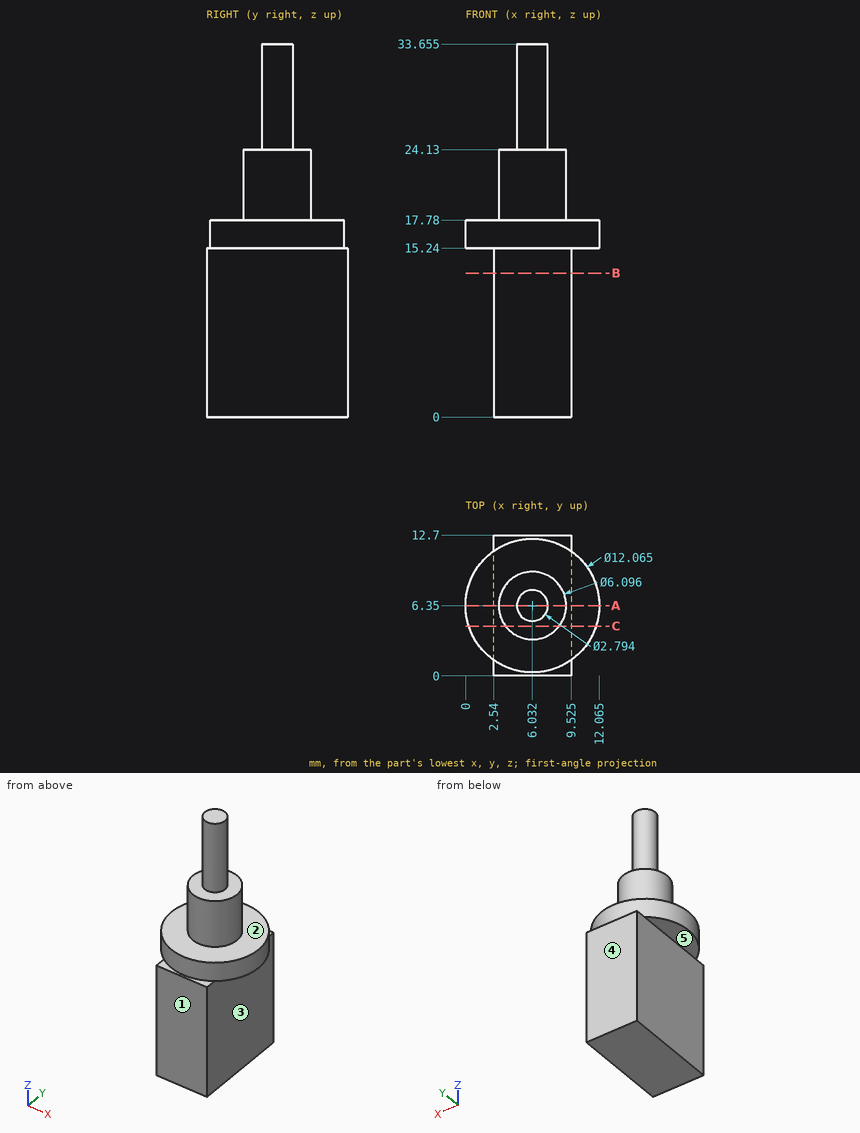
Geometry: see drawing. Coordinates: mm, zero at the bounding-box minimum. A direction names the side the tool comes from. Give positions to 0.01 mm unless a question says otherwise; leave off trailing zeros. Order: outer loops, then holes, each group sorted by start corner. A loop starts at its lowest first (then second) coordinate and runs counter-clockwise, first axis right, second up. Notation, with made-up numbers: M 24,71.25 L 82,71.25 A7 cw 82,83.25 Z; hole C 43,-32 d3. An arc over 180 degrees is marked long. Answer as a JSON object with one key per item and string values.
1. Cut plane B-B, the plane z = 13. Output: boundary loops of the cut face in (x, y) (1 decimal).
Result sheet:
{"outline": "M 2.5,0 L 9.5,0 L 9.5,12.7 L 2.5,12.7 Z"}
2. First-contact query: P1, Ø0.8, axis at x = 1.5, y = 6, coming from the -Z side; P2, Ø1.6, axis at x = 6.5, y = 1, coming from the +Z side; P3, Ø5, axis at x = 9.5, z = 15.5, coming from the -Y side; P4, Ø4, axis at y = 4.5, z = 6.5, coming from the -X side. Flat tips, straight axial feed; report the tip coordinate or a pass-through.
Result sheet:
{"P1": "z = 15.24", "P2": "z = 17.78", "P3": "y = 0", "P4": "x = 2.54"}
3. Ray query, line 1 (Z direction, x = 10, y = 6.75); line 2 (Z direction, x = 3.75, y = 10.25); line 3 (X direction, y = 5.5, z = 6) (1 decimal). Return the intervals inside material, ascending. Write a range as [from, to].
Result sheet:
{"line 1": "[15.24, 17.78]", "line 2": "[0, 17.78]", "line 3": "[2.5, 9.5]"}
4. Cut plane A-A, the plane y = 6.35. Output: boundary loops of the cut face in (x, z) (1 decimal).
Result sheet:
{"outline": "M 0,15.2 L 2.5,15.2 L 2.5,0 L 9.5,0 L 9.5,15.2 L 12.1,15.2 L 12.1,17.8 L 9.1,17.8 L 9.1,24.1 L 7.4,24.1 L 7.4,33.7 L 4.6,33.7 L 4.6,24.1 L 3,24.1 L 3,17.8 L 0,17.8 Z"}
5. Cut plane C-C, the plane y = 4.5. Output: boundary loops of the cut face in (x, z) (1 decimal).
Result sheet:
{"outline": "M 0.3,15.2 L 2.5,15.2 L 2.5,0 L 9.5,0 L 9.5,15.2 L 11.8,15.2 L 11.8,17.8 L 8.5,17.8 L 8.5,24.1 L 3.6,24.1 L 3.6,17.8 L 0.3,17.8 Z"}
6. Reachability of the marked faces 1, 2, 3, 4 and 5 from +Z, -Z, +X, -X, +Y, -Y: full face, straight path, thin tool, end or side. Return the list, or none.
Result sheet:
{"face 1": "+Z, -Z, +X, -X, -Y", "face 2": "+Z", "face 3": "-Z, +X, +Y, -Y", "face 4": "+Z, -Z, +X, -X, +Y", "face 5": "-Z, -X, +Y, -Y"}
